from build123d import *

# Parameters (mm, degrees)
BOSS_EXTRUDE1_DEPTH = 9.525
SKETCH3_R           = 2.15265
CUT_EXTRUDE1_DEPTH  = 37.095993978


with BuildPart() as part:
    # Sketch2 → Boss-Extrude1 (new body)
    with BuildSketch(Plane(origin=(0, 0, 0), x_dir=(1, 0, 0), z_dir=(0, 1, 0))):
        Polygon((-14.2875, 0), (14.2875, 0), (14.2875, 6.35), (5.55625, 6.35), (5.55625, 22.225), (0.79375, 22.225), (0.79375, 31.75), (-3.96875, 31.75), (-3.96875, 6.35), (-14.2875, 6.35), align=None)
    extrude(amount=BOSS_EXTRUDE1_DEPTH)

    # Sketch3 → Cut-Extrude1 (cut, through all)
    with BuildSketch(Plane.XY):
        with Locations((-10.31875, 4.7625)):
            Circle(SKETCH3_R)
        with Locations((10.31875, 4.7625)):
            Circle(SKETCH3_R)
    extrude(amount=-CUT_EXTRUDE1_DEPTH, mode=Mode.SUBTRACT)


solid = part.part
For this review, take the finished solid that the model builds, in its own axes (mm). A direction names the side the tool comes from. Coordinates: 2 decimals unless noted, no trailing zeros. Order: outer loops, then holes, each group sorted by start corner. A loop starts at its lowest first (then second) coordinate and runs counter-clockwise, first axis right, second up. Notation, with made-up numbers: (41, 85.25) - (82, 85.25) arc R35 ccw to (82, 122.25) - close; hole circle Ø9 at (-9.5, 32). An arc over 180 degrees is marked (long way). Answer as CSV lines item,"result". Start each with the question number.
1) Machinability: for faces 4 (the flat face through (0, 5, 0)), 5 (the flat face through (-8, 5, -6.35)), 6 (the flat face through (0.794, 5, -27)), which of the approach directions +Z, -Z, +X, -X, +Y, -Y give a long, thin tool a straight path to every point of the face, cutting with its end or side? Answer none if there is none.
2) Add section D-D (x = 9). State the section outline as (y, z) points (3 decimals), then the cut area to 3 significant figures.
3) Draft analysis for pull direction X (two halves, no side actions). For faces 1 (the flat face through (-2, 5, -31.75)), 2 (the cylindrical face through (-8.266, 5.409, -3.131)), 3 (the flat face through (-14.288, 5, -3)), state which applies: +X half, -X half, draft (parallel to the pull), parting line (faces both ways), or undercut.
4) Add section A-A (x = -10). State the section outline as (y, z) points (3 decimals), then the cut area to 3 significant figures.
5) Add section B-B (y = 5.5). Count the separate pieces of the cut face and the enclosed holes in it, then the cut area to 3 significant figures.
6) Insertion check: P1, Ø1.4, axis at x = 4, y = 4.5, coming from the -Z side (3 decimals); P2, Ø5, axis at x = 10.32, y = 4.76, coming from the -Z side; P3, Ø1.5, axis at y = 5, z = -13, coming from the -X side. Each pin has a flat end and moves straight along its axis. Give the tip position at first contact, or say it passes through.
7) To check wall thickness, follow line 1 along X through (y, z) = (6.5, -2.5); line 2 along X through (y, z) = (1.75, -12.5); line 3 along X through (y, z) = (7.75, -22.5). State the ranges of each line that lie inside material, in increasing order. Write a range as [from, to].
Result:
1,face 4,"+Z, +X, -X, +Y, -Y"
1,face 5,"-Z, -X, +Y, -Y"
1,face 6,"-Z, +X, +Y, -Y"
2,outline,"(0, -6.35) - (3.061, -6.35) - (3.061, 0) - (0, 0) - close; (6.464, -6.35) - (9.525, -6.35) - (9.525, 0) - (6.464, 0) - close"
2,area,"38.9 mm^2"
3,face 1,"draft"
3,face 2,"undercut"
3,face 3,"-X half"
4,outline,"(0, -6.35) - (2.634, -6.35) - (2.634, 0) - (0, 0) - close; (6.891, -6.35) - (9.525, -6.35) - (9.525, 0) - (6.891, 0) - close"
4,area,"33.4 mm^2"
5,separate pieces,"3"
5,enclosed holes,"0"
5,area,"327 mm^2"
6,P1,"z = -22.225"
6,P2,"z = -6.35"
6,P3,"x = -3.97"
7,line 1,"[-14.29, -11.59], [-9.05, 9.05], [11.59, 14.29]"
7,line 2,"[-3.97, 5.56]"
7,line 3,"[-3.97, 0.79]"
